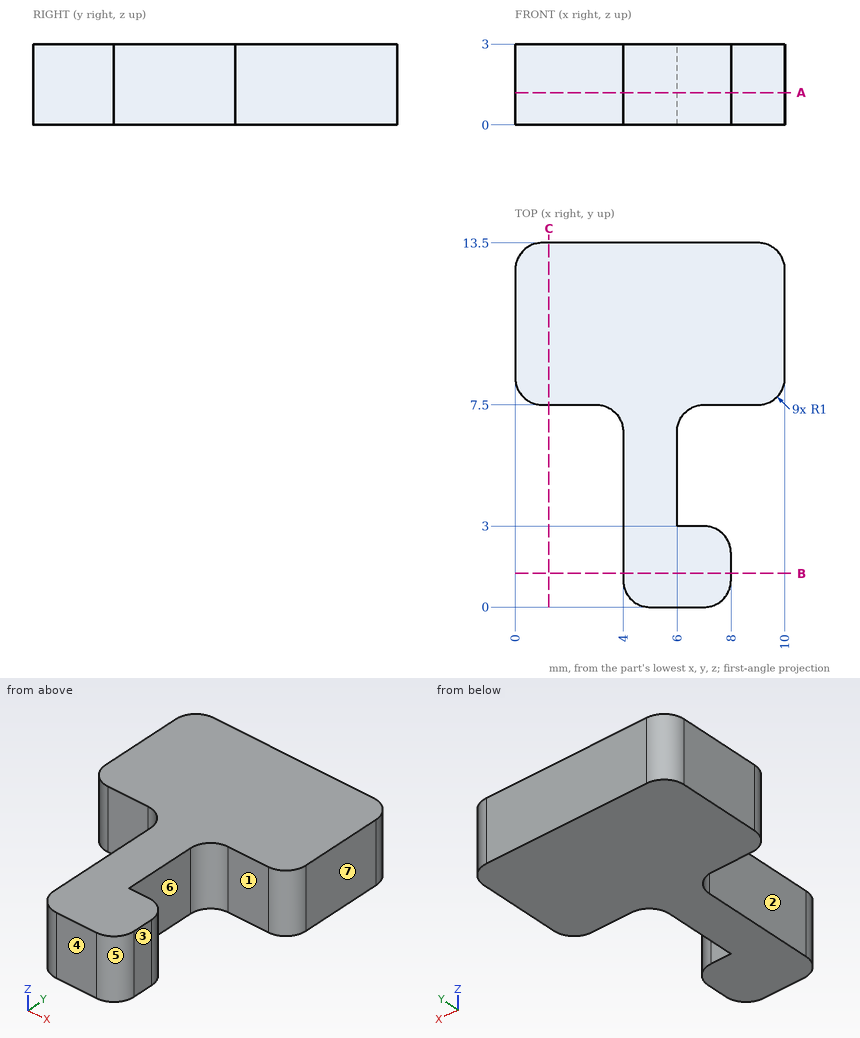
Print and shaded views of the part. All mm, measured from the part's lowest x, y and z. A direction names the side the tool comes from. Give positions to 0.01 mm unless a question says otherwise; leave off trailing zeros. Loops run counter-clockwise (first coordinate to the right, second up) from the corner with the lowest first, then second, coordinate; pieces in that order, holes last. Notation, with made-up numbers: (28.25, 31) -> (37.25, 31) arc R31 ccw to (37.25, 57) -> close; hole circle Ø7 at (18, 37.5). An arc over 180 degrees is marked (long way). Use CSV: the item, a comma, the result in double quotes. Start each with the question number.
1) Slice it at A-A on z = 1.2. Give the cut face in (x, y).
2) Mould opens along Y. For the marked faces 5, 6 and 7 say: released by +Y, released by -Y, zero draft, split by the parting line, or undercut.
3) Flat gauge pins, fed straight in: pin 1 Ø0.6 at (x, z) = (2.5, 1) entering from -Y; pin 2 Ø0.9 at (y, z) = (4, 1.5) entering from -X; pin 3 Ø1.5 at (y, z) = (2, 0.5) entering from +X. Where does each tip first touch, or does it go through?
4) Wall check: line 1 (X direction, y = 4, z = 1.35); line 2 (Y direction, x = 8.5, z = 2); line 3 (X direction, y = 8, z = 1.6). Give the ranges that are in metal, low to high.
5) Tool access for the marked faces 1, 2, 3 and 4: list every direction of +Z, -Z, +X, -X, +Y, -Y with a clear straight run to the whole face (end or side of a thin tool).
6) Slice it at C-C on x = 1.25. Give the cut face in (y, z), plus the area to 3 significant figures.
7) Slice it at B-B on y = 1.25. Give the cut face in (x, z), plus the area to 3 significant figures.
Computed values:
1,outline,"(0, 8.5) arc R1 ccw to (1, 7.5) -> (3, 7.5) arc R1 cw to (4, 6.5) -> (4, 1) arc R1 ccw to (5, 0) -> (7, 0) arc R1 ccw to (8, 1) -> (8, 2) arc R1 ccw to (7, 3) -> (6, 3) -> (6, 6.5) arc R1 cw to (7, 7.5) -> (9, 7.5) arc R1 ccw to (10, 8.5) -> (10, 12.5) arc R1 ccw to (9, 13.5) -> (1, 13.5) arc R1 ccw to (0, 12.5) -> close"
2,face 5,"released by -Y"
2,face 6,"undercut"
2,face 7,"zero draft"
3,pin 1,"stops at y = 7.5"
3,pin 2,"stops at x = 4"
3,pin 3,"stops at x = 8"
4,line 1,"x = 4 to 6"
4,line 2,"y = 7.5 to 13.5"
4,line 3,"x = 0.13 to 9.87"
5,face 1,"+Z, -Z, +X"
5,face 2,"+Z, -Z, -X, -Y"
5,face 3,"+Z, -Z, +X, -Y"
5,face 4,"+Z, -Z, +X, -X, -Y"
6,outline,"(7.5, 0) -> (13.5, 0) -> (13.5, 3) -> (7.5, 3) -> close"
6,area,"18.0 mm^2"
7,outline,"(4, 0) -> (8, 0) -> (8, 3) -> (4, 3) -> close"
7,area,"12.0 mm^2"
